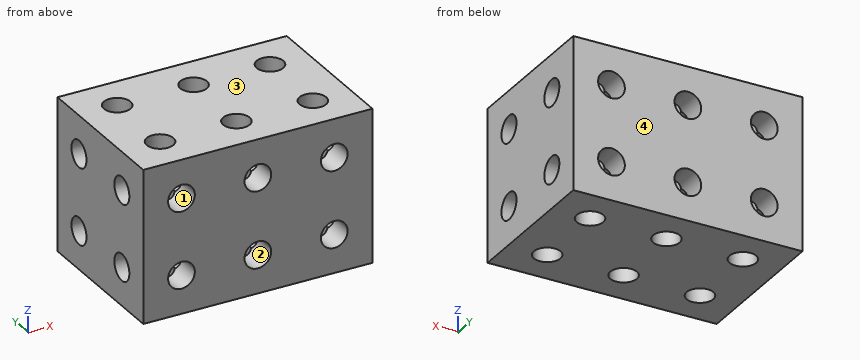
from build123d import *

# Parameters (mm, degrees)
ESQUISSE1_W             = 20
ESQUISSE1_H             = 20
BOSS_EXTRU_1_DEPTH      = 30
ESQUISSE2_R             = 1.75
ENL_V_MAT_EXTRU_1_DEPTH = 42.231056256
ESQUISSE3_R             = 1.75
ENL_V_MAT_EXTRU_2_DEPTH = 40
ESQUISSE4_R             = 1.75
ENL_V_MAT_EXTRU_3_DEPTH = 40


with BuildPart() as part:
    # Esquisse1 → Boss.-Extru.1 (new body)
    with BuildSketch(Plane(origin=(0, 0, 0), x_dir=(0, 0, -1), z_dir=(1, 0, 0))):
        with Locations((10, 10)):
            Rectangle(ESQUISSE1_W, ESQUISSE1_H)
    extrude(amount=BOSS_EXTRU_1_DEPTH)

    # Esquisse2 → Enlèv. mat.-Extru.1 (cut, through all)
    with BuildSketch(Plane(origin=(0, 20, 0), x_dir=(1, 0, 0), z_dir=(0, 1, 0))):
        with Locations(Location((5, 15, 0), (0, 0, 270))):
            Circle(ESQUISSE2_R)
        with Locations(Location((15, 15, 0), (0, 0, 270))):
            Circle(ESQUISSE2_R)
        with Locations(Location((25, 15, 0), (0, 0, 270))):
            Circle(ESQUISSE2_R)
        with Locations((35, 15)):
            Circle(ESQUISSE2_R)
        with Locations(Location((5, 5, 0), (0, 0, 270))):
            Circle(ESQUISSE2_R)
        with Locations(Location((15, 5, 0), (0, 0, 270))):
            Circle(ESQUISSE2_R)
        with Locations(Location((25, 5, 0), (0, 0, 270))):
            Circle(ESQUISSE2_R)
        with Locations((35, 5)):
            Circle(ESQUISSE2_R)
        with Locations((5, -5)):
            Circle(ESQUISSE2_R)
        with Locations((15, -5)):
            Circle(ESQUISSE2_R)
        with Locations((25, -5)):
            Circle(ESQUISSE2_R)
        with Locations((35, -5)):
            Circle(ESQUISSE2_R)
        with Locations((5, -15)):
            Circle(ESQUISSE2_R)
        with Locations((15, -15)):
            Circle(ESQUISSE2_R)
        with Locations((25, -15)):
            Circle(ESQUISSE2_R)
        with Locations((35, -15)):
            Circle(ESQUISSE2_R)
    extrude(amount=-ENL_V_MAT_EXTRU_1_DEPTH, mode=Mode.SUBTRACT)

    # Esquisse3 → Enlèv. mat.-Extru.2 (cut)
    with BuildSketch(Plane.XY):
        with Locations((5, 15)):
            Circle(ESQUISSE3_R)
        with Locations((15, 15)):
            Circle(ESQUISSE3_R)
        with Locations((25, 15)):
            Circle(ESQUISSE3_R)
        with Locations((35, 15)):
            Circle(ESQUISSE3_R)
        with Locations((5, 5)):
            Circle(ESQUISSE3_R)
        with Locations((15, 5)):
            Circle(ESQUISSE3_R)
        with Locations((25, 5)):
            Circle(ESQUISSE3_R)
        with Locations((35, 5)):
            Circle(ESQUISSE3_R)
    extrude(amount=-ENL_V_MAT_EXTRU_2_DEPTH, mode=Mode.SUBTRACT)

    # Esquisse4 → Enlèv. mat.-Extru.3 (cut)
    with BuildSketch(Plane(origin=(30, 0, 0), x_dir=(0, 0, -1), z_dir=(1, 0, 0))):
        with Locations((5, 15)):
            Circle(ESQUISSE4_R)
        with Locations(Location((15, 15, 0), (0, 0, 315))):
            Circle(ESQUISSE4_R)
        with Locations((25, 15)):
            Circle(ESQUISSE4_R)
        with Locations((35, 15)):
            Circle(ESQUISSE4_R)
        with Locations((5, 5)):
            Circle(ESQUISSE4_R)
        with Locations((15, 5)):
            Circle(ESQUISSE4_R)
    extrude(amount=-ENL_V_MAT_EXTRU_3_DEPTH, mode=Mode.SUBTRACT)


solid = part.part
Work out the finished part from the listing and answer in its coordinate system (mm). Face numbers are marked on the shaded views. Round coordinates to 2 decimals unless told otherwise and drop trailing zeros. Loops run counter-clockwise (first coordinate to the right, second up) from the corner with the lowest first, then second, coordinate; pieces in that order, holes last. Notation, with made-up numbers: M -26.75,26 L 31.25,26 A14 cw 31.25,31 Z; hole C 58.25,33.25 d5. An arc over 180 degrees is marked long. One line per question, with ' | ' between items. Start each with the question number.
(1) A cutting plane is placed at C-C on z = -12.25. Write down the section's boundary in (x, y), plus the area to 3 significant figures.
(2) Find the intervals of material crossed by line 1 (Y direction, x = 15, z = -10.25); line 2 (Z direction, x = 25, y = 11); line 3 (X direction, y = 2.8, z = -5), in increasing order.
(3) A cutting plane is placed at A-A on y = 12.25. Write down the section's boundary in (x, z).
(4) For a pull along Z with two mould halves and no side action, classify the marked faces 1, 2, 3 and 4 as released by +Z, released by -Z, zero draft, split by the parting line, or undercut.
(5) A cutting plane is placed at B-B on x = 21.5. Write down the section's boundary in (y, z), plus the area to 3 significant figures.
(6) A cutting plane is placed at D-D on z = -5. Give the number of separate pieces and of enclosed holes in the cut face, plus the area to 4 significant figures.
(7) A flat-ended cylindrical pin translates along its axis: pin 1 Ø2 at (x, y) = (25, 15) entering from -Z. Find the tip coordinate at first contact, or state that the pin passes through.
Geometry check:
1) outline: M 0,0 L 30,0 L 30,20 L 0,20 Z; hole C 5,5 d3.5; hole C 5,15 d3.5; hole C 15,5 d3.5; hole C 15,15 d3.5; hole C 25,5 d3.5; hole C 25,15 d3.5 | area: 542 mm²
2) line 1: y = 0 to 3.25, 6.75 to 13.25, 16.75 to 20 | line 2: z = -20 to -16.75, -13.25 to -6.75, -3.25 to 0 | line 3: x = 0 to 3.25, 6.75 to 13.25, 16.75 to 23.25, 26.75 to 30
3) outline: M 0,-20 L 30,-20 L 30,0 L 0,0 Z; hole C 5,-15 d3.5; hole C 5,-5 d3.5; hole C 15,-15 d3.5; hole C 15,-5 d3.5; hole C 25,-15 d3.5; hole C 25,-5 d3.5
4) face 1: undercut | face 2: undercut | face 3: released by +Z | face 4: zero draft
5) outline: M 0,-20 L 20,-20 L 20,0 L 0,0 Z; hole C 5,-15 d3.5; hole C 5,-5 d3.5; hole C 15,-15 d3.5; hole C 15,-5 d3.5 | area: 362 mm²
6) separate pieces: 12 | enclosed holes: 0 | area: 253.5 mm²
7) pin 1: passes through
